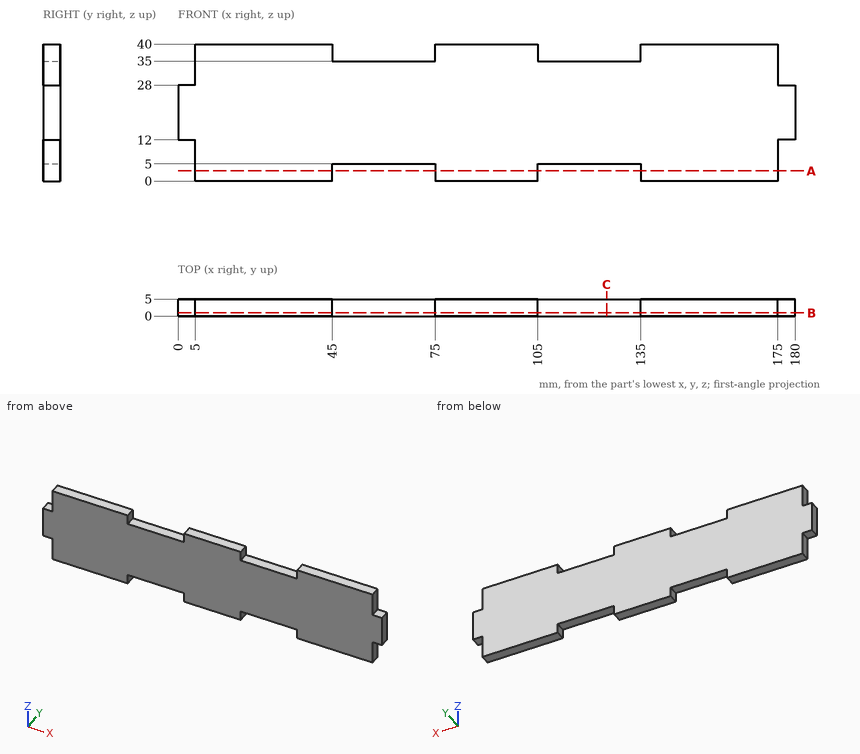
For this review, use the dimensioned drawing (mm, ordinates from the lowest corner) and the shaded views. Round coordinates to 2 decimals unless told otherwise and drop trailing zeros. Write each loop counter-clockwise with the first axis right and the second up, starting at its lowest first coordinate (ties: lowest second). Pieces come first, ordered by that corner, then holes. Notation, with made-up numbers: (43.5, -33) - (84.5, -33) arc R32 ccw to (84.5, 4) - close; hole circle Ø2 at (65.25, -30). An arc over 180 degrees is marked (long way). One line per item, written item: value. Start each with the question number.
1. Consider section C-C on x = 125. Write out the cut boundary in (y, z).
2. Consider section A-A on z = 3. Write out the cut boundary in (x, y).
3. Clearance check with flat-ended pins moving along their axes: P1, Ø8, axis at x = 41, z = 17.5, coming from the -Y side; P2, Ø1.5, axis at x = 178, y = 1.5, coming from the -Z side; P3, Ø2.5, axis at y = 3.5, z = 37, coming from the -X side; P4, Ø2.5, axis at x = 120, y = 3.5, coming from the +Z side. State where each tip first meets the part, or that it passes through.
4. Consider section B-B on y = 1. Write out the cut boundary in (x, z).
5. To check wall thickness, follow L1, parallel to X at y = 1.55, z = 37.5; L2, parallel to Z at x = 47, y = 1.2; L3, parallel to X at y = 0.3, z = 34. State the ranges of each line that lie inside material, in increasing order. Write a range as from..to.
Checks:
1. outline: (0, 5) - (5, 5) - (5, 35) - (0, 35) - close
2. outline: (5, 0) - (45, 0) - (45, 5) - (5, 5) - close; (75, 0) - (105, 0) - (105, 5) - (75, 5) - close; (135, 0) - (175, 0) - (175, 5) - (135, 5) - close
3. P1: stops at y = 0
3. P2: stops at z = 12
3. P3: stops at x = 5
3. P4: stops at z = 35
4. outline: (0, 12) - (5, 12) - (5, 0) - (45, 0) - (45, 5) - (75, 5) - (75, 0) - (105, 0) - (105, 5) - (135, 5) - (135, 0) - (175, 0) - (175, 12) - (180, 12) - (180, 28) - (175, 28) - (175, 40) - (135, 40) - (135, 35) - (105, 35) - (105, 40) - (75, 40) - (75, 35) - (45, 35) - (45, 40) - (5, 40) - (5, 28) - (0, 28) - close
5. L1: x = 5..45, 75..105, 135..175
5. L2: z = 5..35
5. L3: x = 5..175
